The listing builds one solid part. Answer for the finished solid, in the listing's coordinates (mm). Face numbers are marked on the shaded views. A direction names the side the tool comes from. Give positions to 0.01 mm unless a question says otherwise; leave off trailing zeros. Write each loop counter-clockwise with the first axis right and the second up, starting at its lowest first coordinate (ties: lowest second). Pieces come first, ordered by that corner, then holes. Notation, with made-up numbers: (-5.5, 42.5) -> (8.5, 42.5) arc R19 ccw to (8.5, 48.5) -> close; hole circle Ø4 at (62, 52.5). An arc over 180 degrees is marked (long way). One line per question, with ' | ' between items.
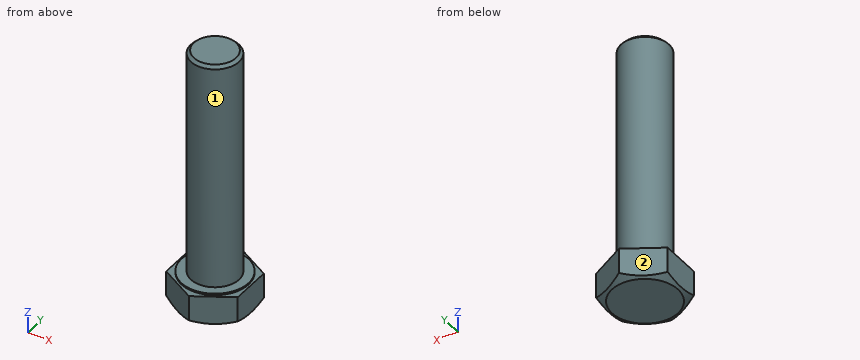
from build123d import *

# Parameters (mm, degrees)
SALIENTE_EXTRUIR1_DEPTH = 10
CROQUIS2_R              = 8.0635
SALIENTE_EXTRUIR2_DEPTH = 77
CROQUIS8_R              = 11.25
SALIENTE_EXTRUIR3_DEPTH = 0.5
CHAFL_N1_SIZE           = 1


with BuildPart() as part:
    # Croquis1 → Saliente-Extruir1 (new body)
    with BuildSketch(Plane.XY):
        Polygon((0, 13.856406461), (-12, 6.92820323), (-12, -6.92820323), (0, -13.856406461), (12, -6.92820323), (12, 6.92820323), align=None)
    extrude(amount=SALIENTE_EXTRUIR1_DEPTH)

    # Croquis2 → Saliente-Extruir2 (add)
    with BuildSketch(Plane.XY.offset(10)):
        Circle(CROQUIS2_R)
    extrude(amount=SALIENTE_EXTRUIR2_DEPTH)

    # Croquis7 → Cortar-Revolución1 (revolve, cut)
    with BuildSketch(Plane(origin=(0, 0, 0), x_dir=(0, 0, -1), z_dir=(1, 0, 0)), mode=Mode.PRIVATE) as cortar_revoluci_n1_sk:
        Polygon((-3.49549265, 17.122750007), (0.466312036, 10.260703002), (0.466312036, 17.122750007), align=None)
    revolve(cortar_revoluci_n1_sk.sketch.rotate(Axis((0, 0, 3.49549265), (0, 0, -1)), 90), axis=Axis((0, 0, 3.49549265), (0, 0, -1)), mode=Mode.SUBTRACT)

    # Croquis8 → Saliente-Extruir3 (add)
    with BuildSketch(Plane.XY.offset(10)):
        Circle(CROQUIS8_R)
    extrude(amount=SALIENTE_EXTRUIR3_DEPTH)

    # Chaflán1
    chafl_n1_edges = [part.edges().sort_by_distance(p)[0] for p in [
        (-8.0635, 0, 87),
    ]]
    chamfer(chafl_n1_edges, length=CHAFL_N1_SIZE)


solid = part.part
Item 1: Find section A-A (y = 0). Write down the section's boundary in (x, z), then the cut area to 3 significant figures.
Answers below:
outline: (-12, 0.54) -> (-11.07, 0) -> (11.07, 0) -> (12, 0.54) -> (12, 10) -> (11.25, 10) -> (11.25, 10.5) -> (8.06, 10.5) -> (8.06, 86) -> (7.06, 87) -> (-7.06, 87) -> (-8.06, 86) -> (-8.06, 10.5) -> (-11.25, 10.5) -> (-11.25, 10) -> (-12, 10) -> close | area: 1,480 mm²
Item 2: Consider line 1 (Z direction, x = -4.75, y = 10); line 2 (Z direction, x = 8.5, y = -8.5); line 3 (Y direction, x = 5.5, z = 42). Determine where each line is inside the solid, lowest interval first. Write a range as [from, to].
Answers below:
line 1: [0, 10.5] | line 2: [0.55, 10] | line 3: [-5.9, 5.9]
Item 3: A tool of negligible diameter and unlimited length cuts with its end or side. For the marked faces 1 and 2, from which of +Z, -Z, +X, -X, +Y, -Y can it reach the whole face along a straight path? Write none if from no direction.
Answers below:
face 1: +Z | face 2: +Z, -Z, -X, +Y
Item 4: Find section B-B (z = 52). Write down the section's boundary in (x, y), then the cut area to 3 significant figures.
Answers below:
outline: circle Ø16.13 at (0, 0) | area: 204 mm²
Item 5: Flat-ended cylindrical pins translate along their axes: pin 1 (12 mm diameter, centred on y = 6.5, z = 44, fed in from -X); pin 2 (5 mm diameter, centred on y = 7.5, z = 54.5, fed in from -X); pin 3 (1.5 mm diameter, centred on x = -5, z = 25.5, fed in from +Y). Find the tip coordinate at first contact, or state that the pin passes through.
Answers below:
pin 1: x = -8.05 | pin 2: x = -6.33 | pin 3: y = 6.85
